Can you work these out from the model? Positions are in its coordinate system, mm. Give positions to 0.01 mm unless a question says otherwise; leave off trailing zeros. Loops run counter-clockwise (first coordinate to the right, second up) from the corner with the lowest first, then second, coordinate; pieces in that order, holes last. Notation, with made-up numbers: (-38, 21) - (-2, 21) arc R10 cw to (-2, 26) - close; hole circle Ø9 at (30.25, 52). An arc over 180 degrees is marked (long way). Use a Markdown table: item, result. Add a question column.
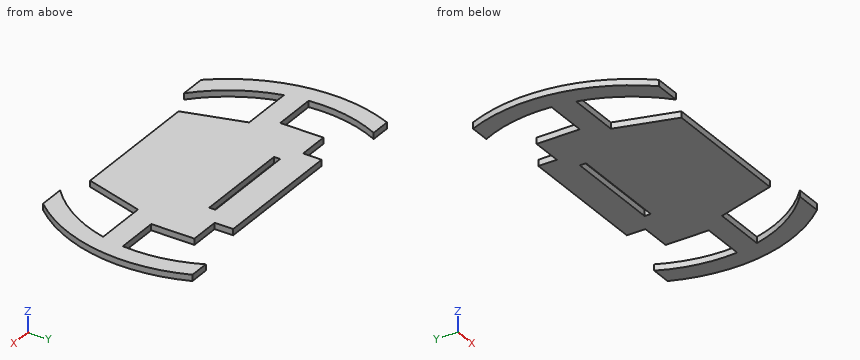
```python
from build123d import *

# Parameters (mm, degrees)
BOSS_EXTRU_1_DEPTH      = 5
ENL_V_MAT_EXTRU_1_DEPTH = 156.951915666
ENL_V_MAT_EXTRU_2_DEPTH = 156.951915666
ESQUISSE7_W             = 10
ESQUISSE7_H             = 42.449970018
ENL_V_MAT_EXTRU_5_DEPTH = 156.951915666
ESQUISSE8_W             = 80
ESQUISSE8_H             = 5
ENL_V_MAT_EXTRU_8_DEPTH = 5


with BuildPart() as part:
    # Esquisse1 → Boss.-Extru.1 (new body)
    with BuildSketch(Plane.XY):
        with BuildLine():
            ThreePointArc((-111.539230767, -28), (-98.317812976, -59.654066514), (-76.347887987, -86))
            Line((-76.347887987, -86), (-97.488460856, -86))
            ThreePointArc((-97.488460856, -86), (-128.254854299, -21.229515978), (-120, 50))
            Line((-120, 50), (-103.561575886, 50))
            ThreePointArc((-103.561575886, 50), (-113.113812186, 20.742841962), (-114.564392374, -10))
            Line((-114.564392374, -10), (-89.564392374, -10))
            Line((-89.564392374, -10), (-89.564392374, 25))
            Line((-89.564392374, 25), (-54.564392374, 25))
            Line((-54.564392374, 25), (-54.564392374, 40))
            Line((-54.564392374, 40), (54.564392374, 40))
            Line((54.564392374, 40), (54.564392374, 25))
            Line((54.564392374, 25), (89.564392374, 25))
            Line((89.564392374, 25), (89.564392374, -10))
            Line((89.564392374, -10), (114.564392374, -10))
            ThreePointArc((114.564392374, -10), (113.113812186, 20.742841962), (103.561575886, 50))
            Line((103.561575886, 50), (120, 50))
            ThreePointArc((120, 50), (128.254854299, -21.229515978), (97.488460856, -86))
            Line((97.488460856, -86), (76.347887987, -86))
            ThreePointArc((76.347887987, -86), (98.317812976, -59.654066514), (111.539230767, -28))
            Line((111.539230767, -28), (68.539230767, -28))
            Line((68.539230767, -28), (54.564392374, -76))
            Line((54.564392374, -76), (-54.564392374, -76))
            Line((-54.564392374, -76), (-68.539230767, -28))
            Line((-68.539230767, -28), (-111.539230767, -28))
        make_face()
    extrude(amount=BOSS_EXTRU_1_DEPTH)

    # Esquisse3 → Enlèv. mat.-Extru.1 (cut, through all)
    with BuildSketch(Plane.XY.offset(5)):
        with BuildLine():
            Line((89.564392374, 25), (79.564392374, 25))
            ThreePointArc((79.564392374, 25), (86.635460186, 22.071067812), (89.564392374, 15))
            Line((89.564392374, 15), (89.564392374, 25))
        make_face()
    extrude(amount=-ENL_V_MAT_EXTRU_1_DEPTH, mode=Mode.SUBTRACT)

    # Esquisse6 → Enlèv. mat.-Extru.2 (cut, through all)
    with BuildSketch(Plane.XY.offset(5)):
        with BuildLine():
            ThreePointArc((-89.564392374, 15), (-86.635460186, 22.071067812), (-79.564392374, 25))
            Line((-79.564392374, 25), (-89.564392374, 25))
            Line((-89.564392374, 25), (-89.564392374, 15))
        make_face()
    extrude(amount=-ENL_V_MAT_EXTRU_2_DEPTH, mode=Mode.SUBTRACT)

    # Esquisse7 → Enlèv. mat.-Extru.5 (cut, through all)
    with BuildSketch(Plane.XY.offset(5)):
        with Locations((-84.564392374, 11.224985009)):
            Rectangle(ESQUISSE7_W, ESQUISSE7_H)
        with Locations((84.564392374, 11.224985009)):
            Rectangle(ESQUISSE7_W, ESQUISSE7_H)
    extrude(amount=-ENL_V_MAT_EXTRU_5_DEPTH, mode=Mode.SUBTRACT)

    # Esquisse8 → Enlèv. mat.-Extru.8 (cut)
    with BuildSketch(Plane.XY.offset(5)):
        with Locations((0, 13.5)):
            Rectangle(ESQUISSE8_W, ESQUISSE8_H)
    extrude(amount=-ENL_V_MAT_EXTRU_8_DEPTH, mode=Mode.SUBTRACT)


solid = part.part
```
1. Will these pins go through, and if not, where does the flat tip stop? P1, Ø2.5, axis at y = 14.5, z = 2, coming from the +X side; P2, Ø1, axis at y = -16.5, z = 1, coming from the +X side; P3, Ø1.5, axis at x = 20, z = 2, coming from the +Y side; P4, Ø6, axis at x = 71, y = -38, coming from the +Z side.
2. Please list where these lines run through material, in increasing order: line 1 along Y through (x, z) = (-34, 3.6); line 2 along X through (y, z) = (12, 3.2); line 3 along X through (y, z) = (20.5, 0.5). Write a range as [from, to].
3. Suppose I cut it at C-C (y = -41.5). List the corners of the cut face in (x, z) for me, and give its area (3 significant figures).
4. Suppose I cut it at A-A (x = 36). List the corners of the cut face in (y, z) for me, and give its area (3 significant figures).
5. Suppose I cut it at B-B (z = 3.3). List the corners of the cut face in (x, y) for me.
6. Suppose I cut it at D-D (y = -67.5). List the corners of the cut face in (x, z) for me.
Results below:
| question | item | result |
|---|---|---|
| 1 | P1 | x = 129.32 |
| 1 | P2 | x = 129.01 |
| 1 | P3 | y = 40 |
| 1 | P4 | through |
| 2 | line 1 | [-76, 11], [16, 40] |
| 2 | line 2 | [-129.44, -114.37], [-79.56, -40], [40, 79.56], [114.37, 129.44] |
| 2 | line 3 | [-128.37, -113.16], [-79.56, 79.56], [113.16, 128.37] |
| 3 | outline | (-123.2, 0) - (-107.25, 0) - (-107.25, 5) - (-123.2, 5) - close; (-64.61, 0) - (64.61, 0) - (64.61, 5) - (-64.61, 5) - close; (107.25, 0) - (123.2, 0) - (123.2, 5) - (107.25, 5) - close |
| 3 | area | 806 mm² |
| 4 | outline | (-76, 0) - (11, 0) - (11, 5) - (-76, 5) - close; (16, 0) - (40, 0) - (40, 5) - (16, 5) - close |
| 4 | area | 555 mm² |
| 5 | outline | (-120, 50) arc R130 ccw to (-97.49, -86) - (-76.35, -86) arc R115 cw to (-111.54, -28) - (-68.54, -28) - (-54.56, -76) - (54.56, -76) - (68.54, -28) - (111.54, -28) arc R115 cw to (76.35, -86) - (97.49, -86) arc R130 ccw to (120, 50) - (103.56, 50) arc R115 cw to (114.56, -10) - (79.56, -10) - (79.56, 25) - (54.56, 25) - (54.56, 40) - (-54.56, 40) - (-54.56, 25) - (-79.56, 25) - (-79.56, -10) - (-114.56, -10) arc R115 cw to (-103.56, 50) - close; hole (-40, 11) - (40, 11) - (40, 16) - (-40, 16) - close |
| 6 | outline | (-111.1, 0) - (-93.11, 0) - (-93.11, 5) - (-111.1, 5) - close; (-57.04, 0) - (57.04, 0) - (57.04, 5) - (-57.04, 5) - close; (93.11, 0) - (111.1, 0) - (111.1, 5) - (93.11, 5) - close |
